```python
from build123d import *

# Parameters (mm, degrees)
SKETCH_1_W      = 100
SKETCH_1_H      = 40
EXTRUDE_1_DEPTH = 10
FILLET_1_R      = 10
EXTRUDE_2_DEPTH = 5


with BuildPart() as part:
    # ｽｹｯﾁ1 → ﾎﾞｽ - 押し出し1 (new body)
    with BuildSketch(Plane(origin=(0, 0, 0), x_dir=(1, 0, 0), z_dir=(0, 1, 0))):
        Rectangle(SKETCH_1_W, SKETCH_1_H)
        with BuildLine():
            Line((44.1, 15.1), (35.9, 15.1))
            ThreePointArc((35.9, 15.1), (35.192893219, 14.807106781), (34.9, 14.1))
            Line((34.9, 14.1), (34.9, 5.9))
            ThreePointArc((34.9, 5.9), (35.192893219, 5.192893219), (35.9, 4.9))
            Line((35.9, 4.9), (44.1, 4.9))
            ThreePointArc((44.1, 4.9), (44.807106781, 5.192893219), (45.1, 5.9))
            Line((45.1, 5.9), (45.1, 14.1))
            ThreePointArc((45.1, 14.1), (44.807106781, 14.807106781), (44.1, 15.1))
        make_face(mode=Mode.SUBTRACT)
        with BuildLine():
            Line((-44.1, 4.9), (-35.9, 4.9))
            ThreePointArc((-35.9, 4.9), (-35.192893219, 5.192893219), (-34.9, 5.9))
            Line((-34.9, 5.9), (-34.9, 14.1))
            ThreePointArc((-34.9, 14.1), (-35.192893219, 14.807106781), (-35.9, 15.1))
            Line((-35.9, 15.1), (-44.1, 15.1))
            ThreePointArc((-44.1, 15.1), (-44.807106781, 14.807106781), (-45.1, 14.1))
            Line((-45.1, 14.1), (-45.1, 5.9))
            ThreePointArc((-45.1, 5.9), (-44.807106781, 5.192893219), (-44.1, 4.9))
        make_face(mode=Mode.SUBTRACT)
        with BuildLine():
            Line((45.1, -5.9), (45.1, -14.1))
            ThreePointArc((45.1, -14.1), (44.807106781, -14.807106781), (44.1, -15.1))
            Line((44.1, -15.1), (35.9, -15.1))
            ThreePointArc((35.9, -15.1), (35.192893219, -14.807106781), (34.9, -14.1))
            Line((34.9, -14.1), (34.9, -5.9))
            ThreePointArc((34.9, -5.9), (35.192893219, -5.192893219), (35.9, -4.9))
            Line((35.9, -4.9), (44.1, -4.9))
            ThreePointArc((44.1, -4.9), (44.807106781, -5.192893219), (45.1, -5.9))
        make_face(mode=Mode.SUBTRACT)
        with BuildLine():
            Line((-44.1, -15.1), (-35.9, -15.1))
            ThreePointArc((-35.9, -15.1), (-35.192893219, -14.807106781), (-34.9, -14.1))
            Line((-34.9, -14.1), (-34.9, -5.9))
            ThreePointArc((-34.9, -5.9), (-35.192893219, -5.192893219), (-35.9, -4.9))
            Line((-35.9, -4.9), (-44.1, -4.9))
            ThreePointArc((-44.1, -4.9), (-44.807106781, -5.192893219), (-45.1, -5.9))
            Line((-45.1, -5.9), (-45.1, -14.1))
            ThreePointArc((-45.1, -14.1), (-44.807106781, -14.807106781), (-44.1, -15.1))
        make_face(mode=Mode.SUBTRACT)
    extrude(amount=EXTRUDE_1_DEPTH)

    # ﾌｨﾚｯﾄ1
    fillet_1_edges = [part.edges().sort_by_distance(p)[0] for p in [
        (50, 5, 20),
        (-50, 5, 20),
        (-50, 5, -20),
        (50, 5, -20),
    ]]
    fillet(fillet_1_edges, radius=FILLET_1_R)

    # ｽｹｯﾁ2 → ﾎﾞｽ - 押し出し2 (add)
    with BuildSketch(Plane(origin=(0, 10, 0), x_dir=(1, 0, 0), z_dir=(0, 1, 0))):
        with BuildLine():
            Line((-9, -10), (9, -10))
            ThreePointArc((9, -10), (9.707106781, -9.707106781), (10, -9))
            Line((10, -9), (10, 9))
            ThreePointArc((10, 9), (9.707106781, 9.707106781), (9, 10))
            Line((9, 10), (-9, 10))
            ThreePointArc((-9, 10), (-9.707106781, 9.707106781), (-10, 9))
            Line((-10, 9), (-10, -9))
            ThreePointArc((-10, -9), (-9.707106781, -9.707106781), (-9, -10))
        make_face()
    extrude(amount=EXTRUDE_2_DEPTH)


solid = part.part
```
Source: CAD feature listing. Evaluate the final solid. Frame: model axes, mm. A direction names the side the tool comes from. Round coordinates to 2 decimals unless told otherwise and drop trailing zeros. Loops run counter-clockwise (first coordinate to the right, second up) from the corner with the lowest first, then second, coordinate; pieces in that order, holes last. Notation, with made-up numbers: M -1,23.5 L 48,23.5 A28 cw 48,48.5 Z; hole C 0,-33 d3. An arc over 180 degrees is marked long. Use a Markdown table: item, result. Add a question column.
1. Section query B-B on x = -2. Return the cut outline in (y, z), then the cut area to 3 significant figures.
2. Mould query, pull axis X, two halves, no side actions, for faces 5 (the flat face through (-1, 0, 0)), 6 (the flat face through (40, 5, 15.1)), 7 (the cylindrical face through (46.99, 5.07, 17.15)). Classes: pulls with the +X half, pulls with the -X half, needs draft (parallel to the pull), parting line crosses it, or undercut.
3. Reachability of faces 1 (the flat face through (45.1, 5, 10)), 2 (the flat face through (-10, 12, 0)), 3 (the flat face through (0, 12, -10)), 4 (the cylindrical face through (-47.15, 5.07, 16.99)) from +Z, -Z, +X, -X, +Y, -Y: full face, straight path, thin tool, end or side. Return the list, or none.
4. Line query: line 1 (Z direction, x = -39.5, y = 3); line 2 (X direction, y = 7.25, z = -5); line 3 (X direction, y = 2.5, z = 12.5). Output: solid intervals per line, ascending.
5. Section query D-D on z = 2. Return the cut outline in (x, y), then the cut area to 3 significant figures.
6. Section query A-A on z = 7. Return the cut outline in (x, y).
7. Section query C-C on y = 2. Give the number of separate pieces and of enclosed holes in the cut face, then the cut area to 3 significant figures.
8. Contact query for flat-ended pins moving along their axis: P1, Ø4, axis at x = -34, z = -10, coming from the +Y side; P2, Ø4, axis at y = 12.5, z = -2, coming from the -X side; P3, Ø5, axis at y = 13.5, z = -5, coming from the +X side. Output: stop coordinate, or through.
Reported:
| question | item | result |
|---|---|---|
| 1 | outline | M 0,-20 L 10,-20 L 10,-10 L 15,-10 L 15,10 L 10,10 L 10,20 L 0,20 Z |
| 1 | area | 500 mm² |
| 2 | face 5 | needs draft |
| 2 | face 6 | undercut |
| 2 | face 7 | pulls with the +X half |
| 3 | face 1 | +Y, -Y |
| 3 | face 2 | +Z, -Z, -X, +Y |
| 3 | face 3 | -Z, +X, -X, +Y |
| 3 | face 4 | +Z, -X, +Y, -Y |
| 4 | line 1 | z = -20 to -15.1, -4.9 to 4.9, 15.1 to 20 |
| 4 | line 2 | x = -50 to -44.54, -35.46 to 35.46, 44.54 to 50 |
| 4 | line 3 | x = -49.68 to -45.1, -34.9 to 34.9, 45.1 to 49.68 |
| 5 | outline | M -50,0 L 50,0 L 50,10 L 10,10 L 10,15 L -10,15 L -10,10 L -50,10 Z |
| 5 | area | 1,100 mm² |
| 6 | outline | M -50,0 L -45.1,0 L -45.1,10 L -50,10 Z; M -34.9,0 L 34.9,0 L 34.9,10 L 10,10 L 10,15 L -10,15 L -10,10 L -34.9,10 Z; M 45.1,0 L 50,0 L 50,10 L 45.1,10 Z |
| 7 | separate pieces | 1 |
| 7 | enclosed holes | 4 |
| 7 | area | 3,500 mm² |
| 8 | P1 | stops at y = 10 |
| 8 | P2 | stops at x = -10 |
| 8 | P3 | stops at x = 10 |
